Can you work these out from the model? Positions are in its coordinate system, mm. A direction names the side the tool comes from. Round coordinates to 2 decimals unless told otherwise and drop trailing zeros. Write each loop counter-clockwise with the first axis right and the second up, starting at its lowest first coordinate (ties: lowest second). Pieces come first, ordered by that corner, then holes. Notation, with made-up numbers: (71.25, 73) -> (130.25, 73) arc R16 cw to (130.25, 82) -> close; hole circle Ø9 at (-7.5, 59.5). An arc over 180 degrees is marked (long way). Write item = value, one per line. Start each with the question number.
1) I'm going to push flat-ended pins straight in: pin 1 (8 mm diameter, centred on x = 9, y = -2, fed in from +Z); pin 2 (4 mm diameter, centred on y = 0, z = 0, fed in from -X); pin 3 (1 mm diameter, centred on x = 13, z = -18, fed in from +Y). Where does each tip first touch, or does it pass through?
2) Imagine slicing it at B-B, the plane y = 31.5. Please give me the cut outline in (x, z), then the cut area to 3 significant figures.
3) Imagine slicing it at C-C, the plane z = 0. Please give me the cut outline in (x, y).
4) Thinking about a two-plate mould opening in Y: for faces 1 (the face through (72.54, -47.15, -46.99)), 2 (the face through (75, 0, 0)), 3 (the face through (82.4, -2.44, 0.54)), 4 (the face through (60, 1, -17)), which applies, +Y half, -Y half, draft (parallel to the pull), parting line (faces both ways), or undercut?
5) Imagine slicing it at D-D, the plane y = -20. Please give me the cut outline in (x, z).
6) Imagine slicing it at A-A, the plane z = -22. Please give me the cut outline in (x, y), then the cut area to 3 significant figures.
7) For faces 5 (the face through (82.395, 1.341, 3.233)), 6 (the face through (72, -1, 50)), which set-ups out of +Z, -Z, +X, -X, +Y, -Y let a thin tool reach every point of the face, with its end or its side?
8) If I drill on line 1 (Y direction, x = 86, z = 0); line 2 (X direction, y = 2.5, z = -21); line 3 (X direction, y = -35, z = 37.5), over which ranges is the centre line in solid material (lowest first)?
from build123d import *

# Parameters (mm, degrees)
SALIENTE_EXTRUIR1_START             = -40
CROQUIS3_R                          = 15
SALIENTE_EXTRUIR1_DEPTH             = 20
SALIENTE_EXTRUIR1_DIRECTION_2_REACH = 93.962
CROQUIS4_W                          = 100
CROQUIS4_H                          = 100
SALIENTE_EXTRUIR2_DEPTH             = 15
REDONDEO1_R                         = 10
REDONDEO2_R                         = 10
CROQUIS5_R                          = 3.5
CROQUIS5_R_2                        = 2.5
SALIENTE_EXTRUIR3_DEPTH             = 15


with BuildPart() as part:
    # Croquis2 → Revolución-Lámina1 (revolve)
    with BuildSketch(Plane.XY):
        with BuildLine():
            ThreePointArc((25, 0), (17.67766953, 17.67766953), (0, 25))
            Line((0, 25), (0, 30))
            ThreePointArc((0, 30), (21.213203436, 21.213203436), (30, 0))
            Line((30, 0), (25, 0))
        make_face()
    revolve(axis=Axis((0, 0, 0), (1, 0, 0)))

    # Croquis3 → Saliente-Extruir1 (add)
    with BuildSketch(Plane.ZY.offset(SALIENTE_EXTRUIR1_START)):
        Circle(CROQUIS3_R)
    extrude(amount=-SALIENTE_EXTRUIR1_DEPTH)

    # Croquis3 → Saliente-Extruir1 direction 2 (add, up to next)
    with BuildSketch(Plane.ZY.offset(SALIENTE_EXTRUIR1_START), mode=Mode.PRIVATE) as saliente_extruir1_direction_2_sk1:
        Circle(CROQUIS3_R)
    saliente_extruir1_direction_2_tool1 = extrude(saliente_extruir1_direction_2_sk1.sketch, amount=SALIENTE_EXTRUIR1_DIRECTION_2_REACH, mode=Mode.PRIVATE) - part.part
    add(saliente_extruir1_direction_2_tool1.solids().sort_by_distance((40, 0, 0))[0])

    # Croquis4 → Saliente-Extruir2 (add)
    with BuildSketch(Plane(origin=(60, 0, 0), x_dir=(0, 0, -1), z_dir=(1, 0, 0))):
        Rectangle(CROQUIS4_W, CROQUIS4_H)
    extrude(amount=SALIENTE_EXTRUIR2_DEPTH)

    # Redondeo1
    redondeo1_edges = [part.edges().sort_by_distance(p)[0] for p in [
        (67.5, -50, -50),
        (67.5, 50, -50),
        (67.5, 50, 50),
        (67.5, -50, 50),
    ]]
    fillet(redondeo1_edges, radius=REDONDEO1_R)

    # Redondeo2
    redondeo2_edges = [part.edges().sort_by_distance(p)[0] for p in [
        (60, 0, -50),
        (60, -50, 0),
        (60, 0, 50),
        (60, 50, 0),
        (60, 47.071067812, -47.071067812),
        (60, 47.071067812, 47.071067812),
        (60, -47.071067812, 47.071067812),
        (60, -47.071067812, -47.071067812),
    ]]
    fillet(redondeo2_edges, radius=REDONDEO2_R)

    # Croquis5 → Saliente-Extruir3 (add)
    with BuildSketch(Plane(origin=(75, 0, 0), x_dir=(0, 0, -1), z_dir=(1, 0, 0))):
        with Locations(Location((0, 0, 0), (0, 0, 180))):
            Circle(CROQUIS5_R)
        Circle(CROQUIS5_R_2, mode=Mode.SUBTRACT)
    extrude(amount=SALIENTE_EXTRUIR3_DEPTH)


solid = part.part
Reported:
q1.pin_1 = 29.54
q1.pin_2 = 24.92
q1.pin_3 = 20.71
q2.outline = (60, -40) arc R10 ccw to (70, -50) -> (75, -50) -> (75, 50) -> (70, 50) arc R10 ccw to (60, 40) -> close
q2.area = 1,460 mm²
q3.outline = (0, -30) arc R30 ccw to (25.98, -15) -> (60, -15) -> (60, -40) arc R10 ccw to (70, -50) -> (75, -50) -> (75, -3.5) -> (90, -3.5) -> (90, -2.5) -> (75, -2.5) -> (75, 2.5) -> (90, 2.5) -> (90, 3.5) -> (75, 3.5) -> (75, 50) -> (70, 50) arc R10 ccw to (60, 40) -> (60, 15) -> (25.98, 15) arc R30 ccw to (0, 30) -> (0, 25) arc R25 cw to (0, -25) -> close
q4.face_1 = -Y half
q4.face_2 = undercut
q4.face_3 = undercut
q4.face_4 = draft
q5.outline = (0, -22.36) arc R22.36 ccw to (0, 22.36) -> (0, 15) arc R15 cw to (0, -15) -> close; (60, -40) arc R10 ccw to (70, -50) -> (75, -50) -> (75, 50) -> (70, 50) arc R10 ccw to (60, 40) -> close
q6.outline = (0, -20.4) arc R20.4 ccw to (0, 20.4) -> (0, 11.87) arc R11.87 cw to (0, -11.87) -> close; (60, -40) arc R10 ccw to (70, -50) -> (75, -50) -> (75, 50) -> (70, 50) arc R10 ccw to (60, 40) -> close
q6.area = 1,890 mm²
q7.face_5 = +X
q7.face_6 = +Z, +X, -X, +Y, -Y
q8.line_1 = -3.5 to -2.5, 2.5 to 3.5
q8.line_2 = 13.33 to 21.28, 60 to 75
q8.line_3 = 60 to 75
